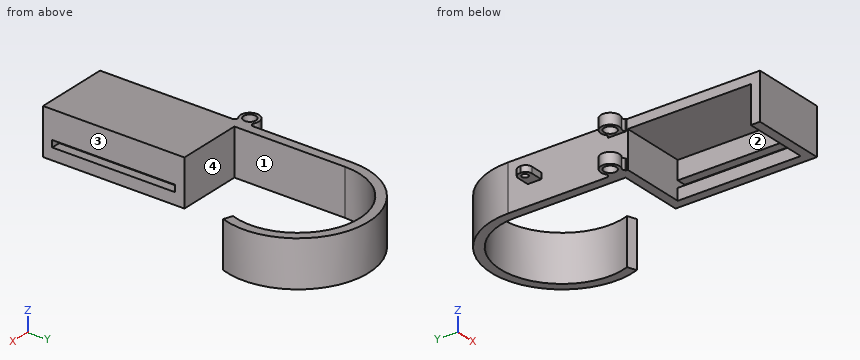
from build123d import *

# Parameters (mm, degrees)
CROQUIS1_W              = 10.6
CROQUIS1_H              = 20
SALIENTE_EXTRUIR1_DEPTH = 1.5
SALIENTE_EXTRUIR2_DEPTH = 7.5
CROQUIS23_W             = 1.1
CROQUIS23_H             = 20
CORTAR_EXTRUIR1_DEPTH   = 25.710524074
SALIENTE_EXTRUIR3_DEPTH = 7.5
CROQUIS25_R             = 1
SALIENTE_EXTRUIR5_DEPTH = 7.5
CROQUIS26_W             = 6.08430057
CROQUIS26_H             = 4
CORTAR_EXTRUIR2_DEPTH   = 7.5
CROQUIS27_W             = 1
CROQUIS27_H             = 2.2
SALIENTE_EXTRUIR6_DEPTH = 3
REDONDEO1_R             = 1
CROQUIS28_R             = 0.5
CORTAR_EXTRUIR3_DEPTH   = 5


with BuildPart() as part:
    # Croquis1 → Saliente-Extruir1 (new body)
    with BuildSketch(Plane.XY):
        with Locations((5.3, 10)):
            Rectangle(CROQUIS1_W, CROQUIS1_H)
    extrude(amount=SALIENTE_EXTRUIR1_DEPTH)

    # Croquis22 → Saliente-Extruir2 (add)
    with BuildSketch(Plane.XY.offset(1.5)):
        Polygon((0, -1.5), (12.1, -1.5), (12.1, 21.5), (0, 21.5), (0, 20), (10.6, 20), (10.6, 0), (0, 0), align=None)
    extrude(amount=-SALIENTE_EXTRUIR2_DEPTH)

    # Croquis23 → Cortar-Extruir1 (cut, through all)
    with BuildSketch(Plane.ZY.offset(-10.6)):
        with Locations((-3.55, 10)):
            Rectangle(CROQUIS23_W, CROQUIS23_H)
    extrude(amount=-CORTAR_EXTRUIR1_DEPTH, mode=Mode.SUBTRACT)

    # Croquis24 → Saliente-Extruir3 (add)
    with BuildSketch(Plane(origin=(0, 0, -6), x_dir=(-1, 0, 0), z_dir=(0, 0, -1))):
        with BuildLine():
            Line((-1.5, 21.5), (-1.5, 39.5))
            ThreePointArc((-1.5, 39.5), (-13.200559707, 49.354344051), (-20.921619337, 36.148419914))
            Line((-20.921619337, 36.148419914), (-22.334862237, 35.645682901))
            ThreePointArc((-22.334862237, 35.645682901), (-13.455643663, 50.832495659), (0, 39.5))
            Line((0, 39.5), (0, 21.5))
            Line((0, 21.5), (-1.5, 21.5))
        make_face()
    extrude(amount=-SALIENTE_EXTRUIR3_DEPTH)

    # Croquis25 → Saliente-Extruir5 (add)
    with BuildSketch(Plane(origin=(0, 0, -6), x_dir=(-1, 0, 0), z_dir=(0, 0, -1))):
        with BuildLine():
            Line((0, 20.21354083), (0, 23.21354083))
            Line((0, 23.21354083), (0.130693606, 23.082847224))
            ThreePointArc((0.130693606, 23.082847224), (0.421244851, 22.940385766), (0.738185248, 23.005685668))
            ThreePointArc((0.738185248, 23.005685668), (3, 21.71354083), (0.738185248, 20.421395992))
            ThreePointArc((0.738185248, 20.421395992), (0.421244851, 20.486695894), (0.130693606, 20.344234436))
            Line((0.130693606, 20.344234436), (0, 20.21354083))
        make_face()
        with Locations((1.5, 21.71354083)):
            Circle(CROQUIS25_R, mode=Mode.SUBTRACT)
    extrude(amount=-SALIENTE_EXTRUIR5_DEPTH)

    # Croquis26 → Cortar-Extruir2 (cut)
    with BuildSketch(Plane.XZ.offset(-20)):
        with Locations((-3.042150285, -2.25)):
            Rectangle(CROQUIS26_W, CROQUIS26_H)
    extrude(amount=-CORTAR_EXTRUIR2_DEPTH, mode=Mode.SUBTRACT)

    # Croquis27 → Saliente-Extruir6 (add)
    with BuildSketch(Plane.ZY):
        with Locations((-2.25, 35.170410703)):
            Rectangle(CROQUIS27_W, CROQUIS27_H)
    extrude(amount=SALIENTE_EXTRUIR6_DEPTH)

    # Redondeo1
    redondeo1_edges = [part.edges().sort_by_distance(p)[0] for p in [
        (-3, 34.070410703, -2.25),
        (-3, 36.270410703, -2.25),
    ]]
    fillet(redondeo1_edges, radius=REDONDEO1_R)

    # Croquis28 → Cortar-Extruir3 (cut)
    with BuildSketch(Plane.XY.offset(-1.75)):
        with Locations((-2, 35.170410703)):
            Circle(CROQUIS28_R)
    extrude(amount=-CORTAR_EXTRUIR3_DEPTH, mode=Mode.SUBTRACT)


solid = part.part
Input: part model. Units: mm. Frame: model coordinates. Face numbers are marked on the shaded views. A direction names the side the tool comes from. Give positions to 0.01 mm unless a question says otherwise; leave off trailing zeros. Loops run counter-clockwise (first coordinate to the right, second up) from the corner with the lowest first, then second, coordinate; pieces in that order, holes last. Notation, with made-up numbers: (-18.75, 24) -> (26.25, 24) arc R26 ccw to (26.25, 47) -> close; hole circle Ø8 at (71, -39.75). An arc over 180 degrees is marked (long way). Answer as a JSON object with one key per item and string values. Group by question number.
Item 1: Cut plane C-C, the plane x = 4.5. Return the cut outline in (y, z).
Item 2: Pin query (flat end, axial travel): P1, Ø2, axis at y = 31.5, z = -2, coming from the +X side; P2, Ø3, axis at x = 3.5, y = 31.5, coming from the +Z side; P3, Ø1, axis at y = 36, z = -1, coming from the -X side; P4, Ø1, axis at y = 9, z = -5, coming from the -X side. Return the tip coordinate at first contact, or that it passes through.
Item 3: Cut plane D-D, the plane z = -4.75. Return the cut outline in (x, y), and give its area (3 significant figures).
Item 4: Cut plane A-A, the plane x = 11.5. Return the cut outline in (y, z).
Item 5: Line query: probe 1 along Y at (x, z) = (11.5, -3.5); probe 2 along Y at (x, z) = (5, -3.5); probe 3 along Y at (x, z) = (11.5, -1.5). Output: solid intervals per line, ascending.
Item 6: Reachability of the marked faces 1, 2, 3 and 4 from +Z, -Z, +X, -X, +Y, -Y: full face, straight path, thin tool, end or side. Return the list, or none.
Item 7: Cut plane B-B, the plane y = 40. Return the cut outline in (x, z), and give its area (3 significant figures).
Checks:
{
 "1": {"outline": "(-1.5, -6) -> (0, -6) -> (0, 0) -> (20, 0) -> (20, -6) -> (21.5, -6) -> (21.5, 1.5) -> (-1.5, 1.5) -> close; (46.64, -6) -> (48.62, -6) -> (48.62, 1.5) -> (46.64, 1.5) -> close"},
 "2": {"P1": "stops at x = 1.5", "P2": "passes through", "P3": "stops at x = 0", "P4": "stops at x = 10.6"},
 "3": {"outline": "(-0.74, 20.42) arc R0.5 cw to (-0.13, 20.34) -> (0, 20.21) -> (0, 20) -> (10.6, 20) -> (10.6, 0) -> (0, 0) -> (0, -1.5) -> (12.1, -1.5) -> (12.1, 21.5) -> (1.5, 21.5) -> (1.5, 39.5) arc R10 cw (long way) to (20.92, 36.15) -> (22.33, 35.65) arc R11.5 ccw (long way) to (0, 39.5) -> (0, 23.21) -> (-0.13, 23.08) arc R0.5 cw to (-0.74, 23.01) arc R1.5 ccw (long way) to start; hole circle Ø2 at (-1.5, 21.71)", "area": "154 mm²"},
 "4": {"outline": "(-1.5, -6) -> (21.5, -6) -> (21.5, 1.5) -> (-1.5, 1.5) -> close; (49.5, -6) -> (51, -6) -> (51, 1.5) -> (49.5, 1.5) -> close; hole (0, -4.1) -> (20, -4.1) -> (20, -3) -> (0, -3) -> close"},
 "5": {"probe 1": "y = -1.5 to 0, 20 to 21.5, 49.5 to 51", "probe 2": "y = -1.5 to 0, 20 to 21.5, 47.1 to 48.99", "probe 3": "y = -1.5 to 21.5, 49.5 to 51"},
 "6": {"face 1": "+Z, -Z", "face 2": "-Z, -X", "face 3": "+Z, -Z, +X, -Y", "face 4": "+Z, -Z, +X"},
 "7": {"outline": "(0.01, -6) -> (1.51, -6) -> (1.51, 1.5) -> (0.01, 1.5) -> close; (21.49, -6) -> (22.99, -6) -> (22.99, 1.5) -> (21.49, 1.5) -> close", "area": "22.5 mm²"}
}
